```python
from build123d import *

# Parameters (mm, degrees)
F0_R            = 27.9
F0_R_2          = 2.2
F0_R_3          = 4.5
F0_R_4          = 1.05
F1_DEPTH        = 3.5
F2_DEPTH        = 1.5
F2_COPIES_COUNT = 26
F3_DEPTH        = 3.5
F3_COPIES_COUNT = 26


# Not quite as in the source:
# - a pattern or mirror of a feature is missing from the dataset's text; its kind, count and spacing are read off the source's solid


with BuildPart() as f1:
    # F0 (on Top) → F1 (new body)
    with BuildSketch(Plane.XY):
        Circle(F0_R)
        with Locations((0, -22.6)):
            Circle(F0_R_2, mode=Mode.SUBTRACT)
        Circle(F0_R_3, mode=Mode.SUBTRACT)
        with Locations((0, -22.6)):
            Circle(F0_R_2)
        with Locations((0, -22.6)):
            Circle(F0_R_4, mode=Mode.SUBTRACT)
        with Locations((0, -22.6)):
            Circle(F0_R_4)
    extrude(amount=-F1_DEPTH)

    # F0 (on Top) → F2 (cut)
    with BuildSketch(Plane.XY):
        with Locations((0, -22.6)):
            Circle(F0_R_2)
        with Locations((0, -22.6)):
            Circle(F0_R_4, mode=Mode.SUBTRACT)
        with Locations((0, -22.6)):
            Circle(F0_R_4)
    f2 = extrude(amount=-F2_DEPTH, mode=Mode.SUBTRACT)

    # F2_copies: F2 ×26 about axis
    f2_copies_axis = Axis((0, 0, 0), (0, 0, 1))
    for i in range(1, F2_COPIES_COUNT):
        add(f2.rotate(f2_copies_axis, i * 360 / F2_COPIES_COUNT), mode=Mode.SUBTRACT)

    # F0 (on Top) → F3 (cut, through all)
    with BuildSketch(Plane.XY):
        with Locations((0, -22.6)):
            Circle(F0_R_4)
    f3 = extrude(amount=-F3_DEPTH, mode=Mode.SUBTRACT)

    # F3_copies: F3 ×26 about axis
    f3_copies_axis = Axis((0, 0, 0), (0, 0, 1))
    for i in range(1, F3_COPIES_COUNT):
        add(f3.rotate(f3_copies_axis, i * 360 / F3_COPIES_COUNT), mode=Mode.SUBTRACT)


solid = f1.part
```
Can you work these out from the model? Positions are in its coordinate system, mm. A direction names the side the tool comes from. Coordinates: 2 decimals unless noted, no trailing zeros. Loops run counter-clockwise (first coordinate to the right, second up) from the corner with the lowest first, then second, coordinate; pieces in that order, holes last. Notation, with made-up numbers: M -17,-8 L 31,-8 A23 ccw 31,20 Z; hole C -26,15.5 d8. An arc over 180 degrees is marked long. Put each result on its own line as item: value. Start each with the question number.
(1) Which directions (+Z, -Z, +X, -X, +Y, -Y) give clear straight access to the entire face, cutting with the end or side of a thin tool? Please do faces 1 (the face through (-24.51, 3.46, -0.74)), 2 (the face through (-17.82, -12.134, -2.486)).
(2) I need wall thicknesses on probe 1 along X at (y, z) = (-1, -1.2); probe 2 along Y at (x, z) = (-11.5, -0.15); probe 3 along X at (y, z) = (3, -1.35). Which ranges of each line are inside material? Lowest first, please.
(3) Imagine slicing it at C-C on x = 15. List the corners of the cut face in (y, z) for me, and give its area (3 significant figures).
(4) Will these pins go through, and if not, where does the flat tip stop? pin 1 Ø1.3 at (x, y) = (-5, -22.5) entering from +Z; pin 2 Ø5.5 at (x, y) = (-5.41, -21.94) entering from -Z; pin 3 Ø1.7 at (x, y) = (10.5, -20.01) entering from -Z.
(5) Imagine slicing it at B-B on z = -2.4. Give the number of separate pieces and of enclosed holes in the cut face, and give its area (3 significant figures).
(6) Imagine slicing it at A-A on x = 0. List the corners of the cut face in (y, z) for me, and give its area (3 significant figures).
Worked answers:
1. face 1: +Z
1. face 2: +Z, -Z
2. probe 1: x = -27.88 to -23.8, -21.07 to -4.39, 4.39 to 21.07, 23.8 to 27.88
2. probe 2: y = -25.42 to -21.97, -18.05 to 18.05, 21.97 to 25.42
2. probe 3: x = -27.74 to -24.62, -20.25 to -3.35, 3.35 to 20.25, 24.62 to 27.74
3. outline: M -23.52,-3.5 L -17.97,-3.5 L -17.97,-1.5 L -19.12,-1.5 L -19.12,0 L -23.52,0 Z; M -15.87,-3.5 L 15.87,-3.5 L 15.87,-1.5 L 14.72,-1.5 L 14.72,0 L -14.72,0 L -14.72,-1.5 L -15.87,-1.5 Z; M 17.97,-3.5 L 23.52,-3.5 L 23.52,0 L 19.12,0 L 19.12,-1.5 L 17.97,-1.5 Z
3. area: 143 mm2
4. pin 1: stops at z = -1.5
4. pin 2: stops at z = -3.5
4. pin 3: passes through
5. separate pieces: 1
5. enclosed holes: 27
5. area: 2,290 mm2
6. outline: M -27.9,-3.5 L -23.65,-3.5 L -23.65,-1.5 L -24.8,-1.5 L -24.8,0 L -27.9,0 Z; M -21.55,-3.5 L -4.5,-3.5 L -4.5,0 L -20.4,0 L -20.4,-1.5 L -21.55,-1.5 Z; M 4.5,-3.5 L 21.55,-3.5 L 21.55,-1.5 L 20.4,-1.5 L 20.4,0 L 4.5,0 Z; M 23.65,-3.5 L 27.9,-3.5 L 27.9,0 L 24.8,0 L 24.8,-1.5 L 23.65,-1.5 Z
6. area: 142 mm2
